The drawing under review shows one solid part. Ordinate dimensions are in mm from its lowest x, y, z. A direction names the side the tool comes from. Coordinates: 2 decimals unless noted, no trailing zeros. Write each loop counter-clockwise with the first axis right and the second up, starting at its lowest first coordinate (ties: lowest second). Pieces come first, ordered by that corner, then holes.
Q1. Add section C-C, the plane x = 42.5. Give the boundary of the cut face in (y, z), plus the area to 3 significant figures.
Q2. Add section B-B, the plane z = 42. Give the boundary of the cut face in (x, y), plus the area to 3 significant figures.
Q3. Machinability: for the marked faces 1, 2, 3 and 4, which of the approach directions +Z, -Z, +X, -X, +Y, -Y give a long, thin tool a straight path to every point of the face, cutting with its end or side? Answer none if there is none.
Q4. Add section D-D, the plane y = 40. Give the boundary of the cut face in (x, z).
Q5. Add section A-A, the plane z = 31. Give the boundary of the cut face in (x, y), plus the area to 3 significant figures.
Q6. Clearance check with flat-ended pins moving along their axes: pin 1 Ø10 at (x, y) = (58, 18) entering from +Z; pin 2 Ø21 at (y, z) = (30, 32) entering from -X; pin 3 Ø2.5 at (x, z) = (4.5, 43) entering from -Y; pin 4 Ø14.5 at (x, y) = (38.5, 22) entering from +Z. State where each tip first meets the part, or that it passes through.
Q7. The part is to be moulded in two halves that separate along X. For the marked faces 5, 6 and 7, say which applies: +X half, -X half, draft (parallel to the pull), parting line (faces both ways), or undercut.
Q8. To check wall thickness, follow probe 1 along X at (y, z) = (3.6, 42); probe 2 along Y at (x, z) = (9, 31); probe 3 along X at (y, z) = (49, 21). State the ranges of each line that lie inside material, in increasing order.
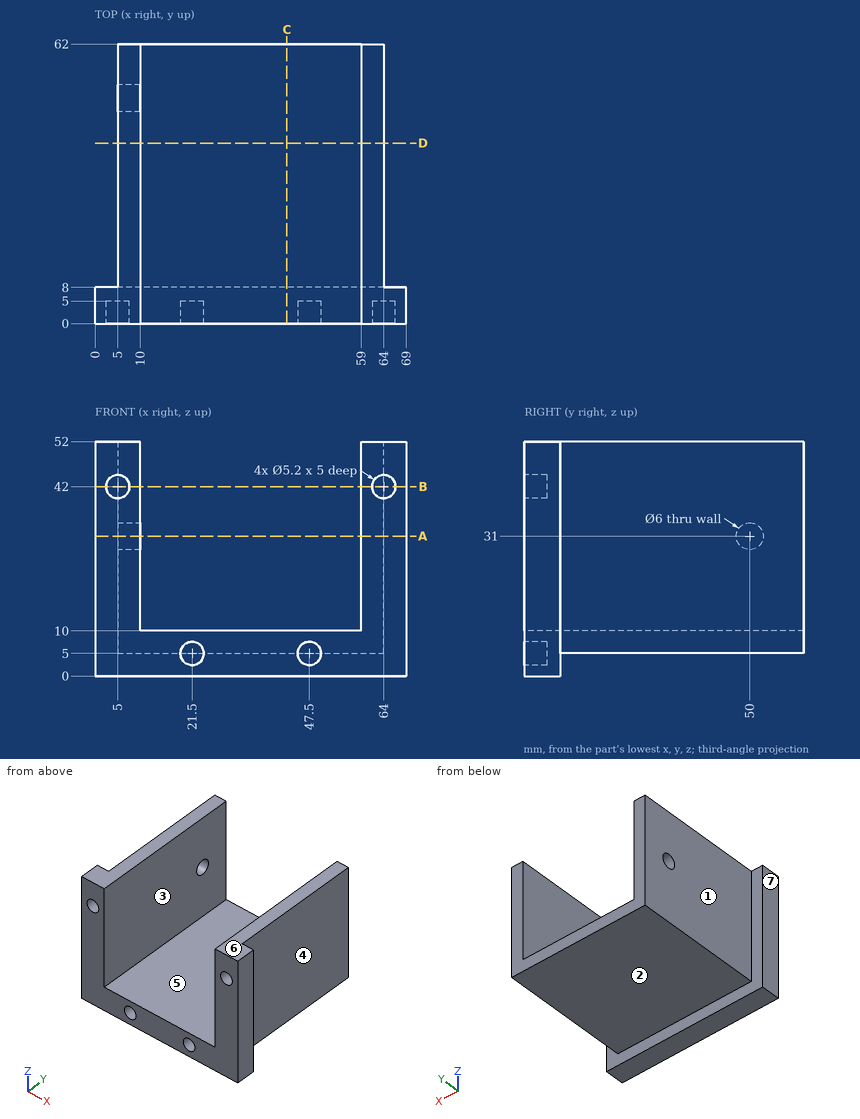
Here are the results:
1. outline: (0, 0) - (8, 0) - (8, 5) - (62, 5) - (62, 10) - (0, 10) - close
1. area: 350 mm2
2. outline: (0, 0) - (2.4, 0) - (2.4, 5) - (7.6, 5) - (7.6, 0) - (10, 0) - (10, 62) - (5, 62) - (5, 8) - (0, 8) - close; (59, 0) - (61.4, 0) - (61.4, 5) - (66.6, 5) - (66.6, 0) - (69, 0) - (69, 8) - (64, 8) - (64, 62) - (59, 62) - close
2. area: 648 mm2
3. face 1: +Z, -Z, -X, +Y
3. face 2: -Z, +X, -X, +Y
3. face 3: +Z, +Y, -Y
3. face 4: +Z, -Z, +X, +Y
4. outline: (5, 5) - (64, 5) - (64, 52) - (59, 52) - (59, 10) - (10, 10) - (10, 52) - (5, 52) - close
5. outline: (0, 0) - (10, 0) - (10, 47) - (5, 47) - (5, 8) - (0, 8) - close; (5, 53) - (10, 53) - (10, 62) - (5, 62) - close; (59, 0) - (69, 0) - (69, 8) - (64, 8) - (64, 62) - (59, 62) - close
5. area: 670 mm2
6. pin 1: stops at z = 52
6. pin 2: stops at x = 5
6. pin 3: stops at y = 5
6. pin 4: stops at z = 10
7. face 5: undercut
7. face 6: draft
7. face 7: -X half
8. probe 1: x = 0 to 2.4, 7.6 to 10, 59 to 61.4, 66.6 to 69
8. probe 2: y = 0 to 47, 53 to 62
8. probe 3: x = 5 to 10, 59 to 64
